from build123d import *

# Parameters (mm, degrees)
F1_DEPTH = 1
F0_W     = 10.6
F0_H     = 20
F2_DEPTH = 7
F3_DEPTH = 11
F4_DEPTH = 16
F5_DEPTH = 8
F6_SIZE2 = 4.99999
F6_SIZE  = 0.19999


# Not quite as in the source:
# - a fillet or chamfer is up to 0.001 mm smaller than in the source, because OpenCascade refuses the exact size


with BuildPart() as f1:
    # F0 (on Top) → F1 (new body)
    with BuildSketch(Plane.XY):
        Polygon((-18.75, 14.5), (-13.25, 14.5), (-13.25, 20), (-10.5, 20), (-10.5, 31), (-21.5, 31), (-21.5, 20), (-18.75, 20), align=None)
    extrude(amount=F1_DEPTH)



with BuildPart() as f1b:
    # F0 (on Top) → F1, piece 2 (new body)
    with BuildSketch(Plane.XY):
        Polygon((5.5, 31), (-5.5, 31), (-5.5, 20), (-2.75, 20), (-2.75, 14.5), (2.75, 14.5), (2.75, 20), (5.5, 20), align=None)
    extrude(amount=F1_DEPTH)


with BuildPart() as f1c:
    # F0 (on Top) → F1, piece 3 (new body)
    with BuildSketch(Plane.XY):
        Polygon((21.5, 31), (10.5, 31), (10.5, 20), (13.25, 20), (13.25, 14.5), (18.75, 14.5), (18.75, 20), (21.5, 20), align=None)
    extrude(amount=F1_DEPTH)


with BuildPart() as f2:
    # F0 (on Top) → F2 (new body)
    with BuildSketch(Plane.XY):
        with Locations((-18, 3.5)):
            Rectangle(F0_W, F0_H)
    extrude(amount=F2_DEPTH)


with BuildPart() as f2b:
    # F0 (on Top) → F2, piece 2 (new body)
    with BuildSketch(Plane.XY):
        with Locations((-6, 3.5)):
            Rectangle(F0_W, F0_H)
    extrude(amount=F2_DEPTH)


with BuildPart() as f2c:
    # F0 (on Top) → F2, piece 3 (new body)
    with BuildSketch(Plane.XY):
        with Locations((6, 3.5)):
            Rectangle(F0_W, F0_H)
    extrude(amount=F2_DEPTH)


with BuildPart() as f2d:
    # F0 (on Top) → F2, piece 4 (new body)
    with BuildSketch(Plane.XY):
        with Locations((18, 3.5)):
            Rectangle(F0_W, F0_H)
    extrude(amount=F2_DEPTH)


with BuildPart() as f3:
    # F0 (on Top) → F3 (new body)
    with BuildSketch(Plane.XY):
        Polygon((-18, -8), (-23.25, -13), (-23.25, -20.5), (-12.75, -20.5), (-12.75, -13), align=None)
    extrude(amount=F3_DEPTH)


with BuildPart() as f3b:
    # F0 (on Top) → F3, piece 2 (new body)
    with BuildSketch(Plane.XY):
        Polygon((-5.25, -13), (-5.25, -20.5), (5.25, -20.5), (5.25, -13), (0, -8), align=None)
    extrude(amount=F3_DEPTH)


with BuildPart() as f3c:
    # F0 (on Top) → F3, piece 3 (new body)
    with BuildSketch(Plane.XY):
        Polygon((12.75, -13), (12.75, -20.5), (23.25, -20.5), (23.25, -13), (18, -8), align=None)
    extrude(amount=F3_DEPTH)


with BuildPart() as f3d:
    # F0 (on Top) → F3, piece 4 (new body)
    with BuildSketch(Plane.XY):
        Polygon((14.25, -31.5), (14.25, -24), (9, -19), (3.75, -24), (3.75, -31.5), align=None)
    extrude(amount=F3_DEPTH)


with BuildPart() as f3e:
    # F0 (on Top) → F3, piece 5 (new body)
    with BuildSketch(Plane.XY):
        Polygon((-3.75, -31.5), (-3.75, -24), (-9, -19), (-14.25, -24), (-14.25, -31.5), align=None)
    extrude(amount=F3_DEPTH)


with BuildPart() as f1_1:
    add(f1.part)

    add(f1b.part)  # F4 merges F1b

    add(f1c.part)  # F4 merges F1c

    add(f2.part)  # F4 merges F2

    add(f2b.part)  # F4 merges F2b

    add(f2c.part)  # F4 merges F2c

    add(f2d.part)  # F4 merges F2d

    add(f3.part)  # F4 merges F3

    add(f3b.part)  # F4 merges F3b

    add(f3c.part)  # F4 merges F3c

    add(f3d.part)  # F4 merges F3d

    add(f3e.part)  # F4 merges F3e
    # F0 (on Top) → F4 (join)
    with BuildSketch(Plane.XY):
        with BuildLine():
            ThreePointArc((24.3, 28.5), (23.0405591591, 31.5405591591), (20, 32.8))
            Line((20, 32.8), (-20, 32.8))
            ThreePointArc((-20, 32.8), (-23.0405591591, 31.5405591591), (-24.3, 28.5))
            Line((-24.3, 28.5), (-24.3, -28.5))
            ThreePointArc((-24.3, -28.5), (-23.0405591591, -31.5405591591), (-20, -32.8))
            Line((-20, -32.8), (20, -32.8))
            ThreePointArc((20, -32.8), (23.0405591591, -31.5405591591), (24.3, -28.5))
            Line((24.3, -28.5), (24.3, 28.5))
        make_face()
        Polygon((-9, -19), (-3.75, -24), (-3.75, -31.5), (-14.25, -31.5), (-14.25, -24), align=None, mode=Mode.SUBTRACT)
        Polygon((-23.25, -20.5), (-23.25, -13), (-18, -8), (-12.75, -13), (-12.75, -20.5), align=None, mode=Mode.SUBTRACT)
        Polygon((9, -19), (14.25, -24), (14.25, -31.5), (3.75, -31.5), (3.75, -24), align=None, mode=Mode.SUBTRACT)
        Polygon((5.25, -20.5), (-5.25, -20.5), (-5.25, -13), (0, -8), (5.25, -13), align=None, mode=Mode.SUBTRACT)
        Polygon((23.25, -20.5), (12.75, -20.5), (12.75, -13), (18, -8), (23.25, -13), align=None, mode=Mode.SUBTRACT)
        with Locations((-18, 3.5)):
            Rectangle(F0_W, F0_H, mode=Mode.SUBTRACT)
        with Locations((-6, 3.5)):
            Rectangle(F0_W, F0_H, mode=Mode.SUBTRACT)
        Polygon((-13.25, 20), (-13.25, 14.5), (-18.75, 14.5), (-18.75, 20), (-21.5, 20), (-21.5, 31), (-10.5, 31), (-10.5, 20), align=None, mode=Mode.SUBTRACT)
        with Locations((6, 3.5)):
            Rectangle(F0_W, F0_H, mode=Mode.SUBTRACT)
        with Locations((18, 3.5)):
            Rectangle(F0_W, F0_H, mode=Mode.SUBTRACT)
        Polygon((-5.5, 20), (-5.5, 31), (5.5, 31), (5.5, 20), (2.75, 20), (2.75, 14.5), (-2.75, 14.5), (-2.75, 20), align=None, mode=Mode.SUBTRACT)
        Polygon((10.5, 20), (10.5, 31), (21.5, 31), (21.5, 20), (18.75, 20), (18.75, 14.5), (13.25, 14.5), (13.25, 20), align=None, mode=Mode.SUBTRACT)
    extrude(amount=F4_DEPTH)

    # F0 (on Top) → F5 (join)
    with BuildSketch(Plane.XY):
        with BuildLine():
            ThreePointArc((25, 28.5), (23.5355339059, 32.0355339059), (20, 33.5))
            Line((20, 33.5), (-20, 33.5))
            ThreePointArc((-20, 33.5), (-23.5355339059, 32.0355339059), (-25, 28.5))
            Line((-25, 28.5), (-25, -28.5))
            ThreePointArc((-25, -28.5), (-23.5355339059, -32.0355339059), (-20, -33.5))
            Line((-20, -33.5), (20, -33.5))
            ThreePointArc((20, -33.5), (23.5355339059, -32.0355339059), (25, -28.5))
            Line((25, -28.5), (25, 28.5))
        make_face()
        with BuildLine():
            Line((-20, 32.8), (20, 32.8))
            ThreePointArc((20, 32.8), (23.0405591591, 31.5405591591), (24.3, 28.5))
            Line((24.3, 28.5), (24.3, -28.5))
            ThreePointArc((24.3, -28.5), (23.0405591591, -31.5405591591), (20, -32.8))
            Line((20, -32.8), (-20, -32.8))
            ThreePointArc((-20, -32.8), (-23.0405591591, -31.5405591591), (-24.3, -28.5))
            Line((-24.3, -28.5), (-24.3, 28.5))
            ThreePointArc((-24.3, 28.5), (-23.0405591591, 31.5405591591), (-20, 32.8))
        make_face(mode=Mode.SUBTRACT)
    extrude(amount=F5_DEPTH)

    # F6 (size 0.2 and 5 in the source; OpenCascade refuses exactly that, so slightly less here)
    f6_edges = [f1_1.edges().sort_by_distance(p)[0] for p in [
        (23.040559, 31.540559, 16),
        (0, 32.8, 16),
        (-23.040559, 31.540559, 16),
        (-24.3, 0, 16),
        (-23.040559, -31.540559, 16),
        (0, -32.8, 16),
        (23.040559, -31.540559, 16),
        (24.3, 0, 16),
        (-6.375, -21.5, 16),
        (-3.75, -27.75, 16),
        (-9, -31.5, 16),
        (-14.25, -27.75, 16),
        (-11.625, -21.5, 16),
        (-23.25, -16.75, 16),
        (-20.625, -10.5, 16),
        (-15.375, -10.5, 16),
        (-12.75, -16.75, 16),
        (-18, -20.5, 16),
        (11.625, -21.5, 16),
        (14.25, -27.75, 16),
        (9, -31.5, 16),
        (3.75, -27.75, 16),
        (6.375, -21.5, 16),
        (0, -20.5, 16),
        (-5.25, -16.75, 16),
        (-2.625, -10.5, 16),
        (2.625, -10.5, 16),
        (5.25, -16.75, 16),
        (18, -20.5, 16),
        (12.75, -16.75, 16),
        (15.375, -10.5, 16),
        (20.625, -10.5, 16),
        (23.25, -16.75, 16),
        (-23.3, 3.5, 16),
        (-18, 13.5, 16),
        (-12.7, 3.5, 16),
        (-18, -6.5, 16),
        (-6, -6.5, 16),
        (-11.3, 3.5, 16),
        (-6, 13.5, 16),
        (-0.7, 3.5, 16),
        (-13.25, 17.25, 16),
        (-16, 14.5, 16),
        (-18.75, 17.25, 16),
        (-20.125, 20, 16),
        (-21.5, 25.5, 16),
        (-16, 31, 16),
        (-10.5, 25.5, 16),
        (-11.875, 20, 16),
        (6, -6.5, 16),
        (0.7, 3.5, 16),
        (6, 13.5, 16),
        (11.3, 3.5, 16),
        (18, -6.5, 16),
        (12.7, 3.5, 16),
        (18, 13.5, 16),
        (23.3, 3.5, 16),
        (-5.5, 25.5, 16),
        (0, 31, 16),
        (5.5, 25.5, 16),
        (4.125, 20, 16),
        (2.75, 17.25, 16),
        (0, 14.5, 16),
        (-2.75, 17.25, 16),
        (-4.125, 20, 16),
        (10.5, 25.5, 16),
        (16, 31, 16),
        (21.5, 25.5, 16),
        (20.125, 20, 16),
        (18.75, 17.25, 16),
        (16, 14.5, 16),
        (13.25, 17.25, 16),
        (11.875, 20, 16),
    ]]
    f6_side = f1_1.faces().sort_by_distance((0, -2.524734, 16))[0]
    chamfer(f6_edges, length=F6_SIZE, length2=F6_SIZE2, reference=f6_side)


solid = f1_1.part
Here's how the part is built. I have some questions about the finished solid (model axes, mm). Coordinates: 2 decimals unless noted, no trailing zeros. Write each loop counter-clockwise with the first axis right and the second up, starting at its lowest first coordinate (ties: lowest second). Pieces come first, ordered by that corner, then holes.
Item 1: If I drill on line 1 (X direction, y = 4, z = 9); line 2 (X direction, y = 26, z = 5.5); line 3 (Y direction, x = 22.5, z = 15.75), over which ranges is the centre line in solid material (lowest first)?
Item 2: Will these pins go through, and if not, where does the flat tip stop? pin 1 (1.5 mm diameter, centred on y = 11.5, z = 9, fed in from -X); pin 2 (1 mm diameter, centred on y = 20, z = 12, fed in from +X); pin 3 (3 mm diameter, centred on y = 6.5, z = 8.5, fed in from -X); pin 4 (1 mm diameter, centred on y = -20, z = 14.5, fed in from -X).
Item 3: I want a section at B-B on y = 16. Write out the boundary of the cut face in (x, z), and give its area (3 significant figures).
Item 4: If we mould it in two halves opening along Y, with no side actions, what happens to faces 1 (the flat face through (0.3, 32.7, 13.5)), 2 (the flat face through (-11.693, -21.429, 13.465)), 3 (the flat face through (-4, 20, 6)), 4 (the cylindrical face through (23.5, -32.07, 3.94))? For each: +Y half, -Y half, draft (parallel to the pull), parting line (faces both ways), or undercut.
Item 5: I want a section at A-A on z = 2.25. Count the separate pieces of the cut face and the enclosed holes in it, and give its area (3 significant figures).
Findings below:
1. line 1: x = -24.3 to -23.3, -12.7 to -11.3, -0.7 to 0.7, 11.3 to 12.7, 23.3 to 24.3
1. line 2: x = -25 to -21.5, -10.5 to -5.5, 5.5 to 10.5, 21.5 to 25
1. line 3: y = -31.76 to -20.69, -12.02 to -6.69, 13.69 to 31.76
2. pin 1: stops at x = -24.3
2. pin 2: stops at x = 24.28
2. pin 3: stops at x = -25
2. pin 4: stops at x = -24.18
3. outline: (-25, 0) - (25, 0) - (25, 8) - (24.3, 8) - (24.3, 11) - (24.1, 16) - (18.95, 16) - (18.75, 11) - (18.75, 1) - (13.25, 1) - (13.25, 11) - (13.05, 16) - (2.95, 16) - (2.75, 11) - (2.75, 1) - (-2.75, 1) - (-2.75, 11) - (-2.95, 16) - (-13.05, 16) - (-13.25, 11) - (-13.25, 1) - (-18.75, 1) - (-18.75, 11) - (-18.95, 16) - (-24.1, 16) - (-24.3, 11) - (-24.3, 8) - (-25, 8) - close
3. area: 537 mm2
4. face 1: +Y half
4. face 2: undercut
4. face 3: undercut
4. face 4: -Y half
5. separate pieces: 1
5. enclosed holes: 3
5. area: 2,870 mm2
